Check sheet for the drawn part. Datum: minimum x, y, z corner. Units: mm. Round coordinates to 2 decimals unless told otherwise and drop trailing zeros. Write each loop counter-clockwise with the first axis right and the second up, starting at its lowest first coordinate (ties: lowest second). Pieces come first, ordered by that corner, then holes. Notation, with made-up numbers: M -26.75,0 L -7.75,0 A22 ccw -7.75,12 Z; hole C 45.25,50 d11. An arc over 180 degrees is marked long. Put each result on its own line as item: value.
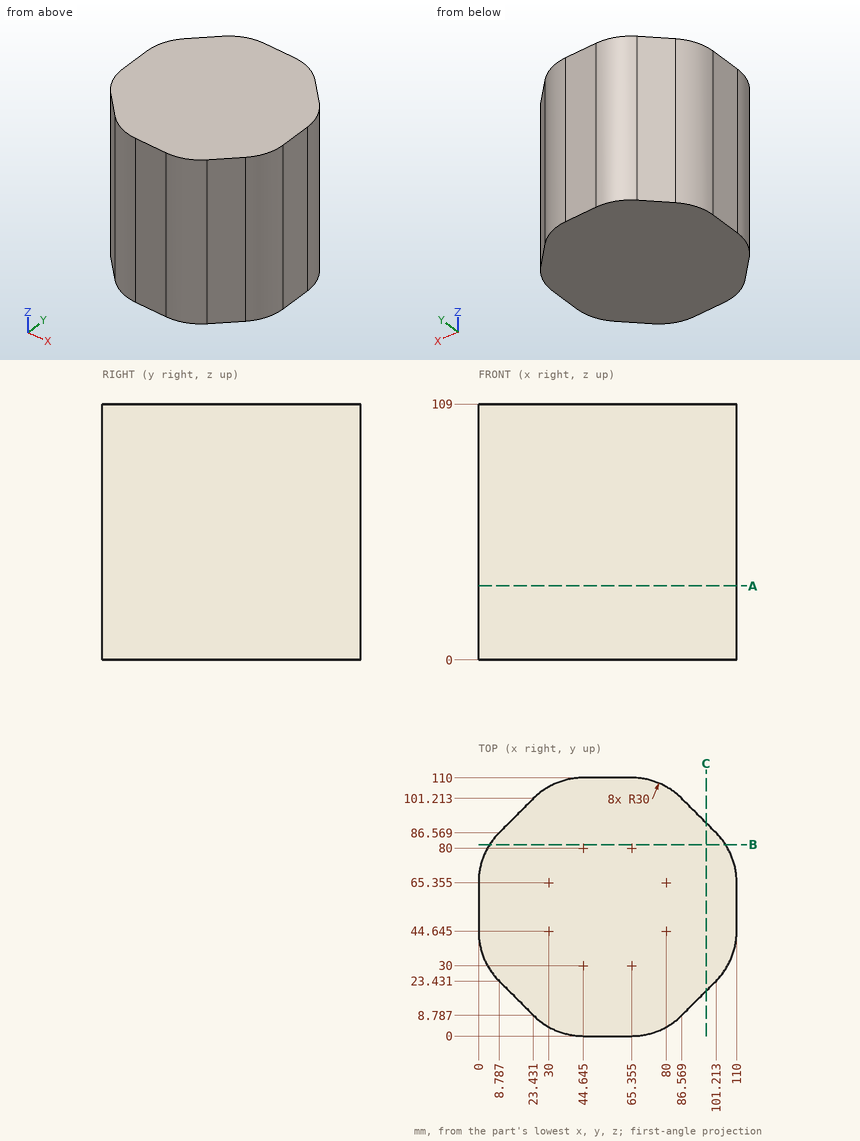
1. Cross-section at B-B (y = 81.5). Enter the section's corners in (x, z) (1 decimal).
Computed values:
outline: M 4.7,0 L 105.3,0 L 105.3,109 L 4.7,109 Z
2. Depth check by flat-ended pin: pin 1 Ø10 at (x, z) = (23.5, 73.5) entering from -Y (1 decimal); pin 2 Ø1 at (y, z) = (88.5, 31.5) entering from -X; pin 3 Ø2 at (x, z) = (43.5, 11) entering from +Y. Enter the tip coordinate at first touch or a pass-through.
Computed values:
pin 1: stops at y = 4.7
pin 2: stops at x = 10.22
pin 3: stops at y = 110
3. Cross-section at C-C (x = 97). Enter the section's corners in (y, z).
Computed values:
outline: M 19.22,0 L 90.78,0 L 90.78,109 L 19.22,109 Z
4. Scan lines: probe 1 along X at (y, z) = (43.5, 93); probe 2 along X at (y, z) = (100.5, 52); probe 3 along Y at (x, z) = (41.5, 63) (1 decimal). Record each from-to range of solid material in increasing order.
Computed values:
probe 1: x = 0.02 to 109.98
probe 2: x = 22.72 to 87.28
probe 3: y = 0.2 to 109.8
5. Cross-section at A-A (z = 31.5). Enter the section's corners in (x, y) (1 decimal), then the cut area to 3 significant figures.
Computed values:
outline: M 0,44.6 A30 ccw 8.8,23.4 L 23.4,8.8 A30 ccw 44.6,0 L 65.4,0 A30 ccw 86.6,8.8 L 101.2,23.4 A30 ccw 110,44.6 L 110,65.4 A30 ccw 101.2,86.6 L 86.6,101.2 A30 ccw 65.4,110 L 44.6,110 A30 ccw 23.4,101.2 L 8.8,86.6 A30 ccw 0,65.4 Z
area: 9,870 mm2
